from build123d import *

# Parameters (mm, degrees)
SKETCH2_R           = 10.30551588
SKETCH2_W           = 5
SKETCH2_H           = 3
BOSS_EXTRUDE1_DEPTH = 3


# Read off the part's stored shape, not the designer's step: Gear 60pitch part02.STEP
with BuildPart() as part:
    # Sketch2 → Boss-Extrude1 (new body)
    with BuildSketch(Plane.XY.offset(1)):
        Circle(SKETCH2_R)
        Rectangle(SKETCH2_W, SKETCH2_H, mode=Mode.SUBTRACT)
    extrude(amount=BOSS_EXTRUDE1_DEPTH)


solid = part.part
Work out the finished part from the listing and answer in its coordinate system (mm). A direction names the side the tool comes from. Coordinates: 2 decimals unless noted, no trailing zeros. Write each loop counter-clockwise with the first axis right and the second up, starting at its lowest first coordinate (ties: lowest second). Pieces come first, ordered by that corner, then holes. Notation, with made-up numbers: M 76,73 L 80,73 A15 ccw 80,102 Z; hole C 37,-10.75 d1. An arc over 180 degrees is marked long. Use one line per item in the form item = value. Start each with the question number.
1. A tool of negligible diameter and unlimited length cuts with its end or side. For faces 5 (the face through (0, -2, 4)), 6 (the face through (2.5, 0, 2)), from which of +Z, -Z, +X, -X, +Y, -Y can it reach the whole face along a straight path? Write none if from no direction.
2. The part is cut by section B-B (x = 0). Give the vertices of the cut face in (y, z).
3. Each of these flat-tipped pins is pushed along its axis until it touches: P1, Ø1, axis at x = 6, z = 3, coming from the -Y side; P2, Ø0.9, axis at x = 1, z = 2, coming from the -Y side. Where does it stop, or does it pass through?
4. Straight lines are drawn through the part: probe 1 along Y at (x, z) = (0, 3.4); probe 2 along X at (y, z) = (-1, 2.4); probe 3 along Y at (x, z) = (-5.25, 3.5). For each, find the intervals that lie inside material, in ascending order. Write a range as from..to.
5. The part is cut by section C-C (z = 2). Give the vertices of the cut face in (x, y), plus the area to 3 significant figures.
6. The part is cut by section A-A (y = 0). Give the vertices of the cut face in (x, z), plus the area to 3 significant figures.
7. The part is cut by section D-D (x = 5). Give the vertices of the cut face in (y, z).
8. The mould has two halves that part along X. Classify faces 1 (the face through (0, -2, 1)), 2 (the face through (-2.5, 0, 2)), 3 (the face through (0, 1.5, 2)), 4 (the face through (-10.296, 0.453, 2.479)): released by +X, released by -X, zero draft, split by the parting line, or undercut.
Evaluation:
q1.face_5 = +Z, +X, -X, +Y, -Y
q1.face_6 = +Z, -Z
q2.outline = M -10.31,1 L -1.5,1 L -1.5,4 L -10.31,4 Z; M 1.5,1 L 10.31,1 L 10.31,4 L 1.5,4 Z
q3.P1 = -8.72
q3.P2 = -10.29
q4.probe_1 = -10.31..-1.5, 1.5..10.31
q4.probe_2 = -10.26..-2.5, 2.5..10.26
q4.probe_3 = -8.87..8.87
q5.outline = C 0,0 d20.61; hole M -2.5,-1.5 L 2.5,-1.5 L 2.5,1.5 L -2.5,1.5 Z
q5.area = 319 mm^2
q6.outline = M -10.31,1 L -2.5,1 L -2.5,4 L -10.31,4 Z; M 2.5,1 L 10.31,1 L 10.31,4 L 2.5,4 Z
q6.area = 46.8 mm^2
q7.outline = M -9.01,1 L 9.01,1 L 9.01,4 L -9.01,4 Z
q8.face_1 = zero draft
q8.face_2 = undercut
q8.face_3 = undercut
q8.face_4 = split by the parting line
